Geometry check sheet. Reference: the model listing, model coordinates, mm. Face numbers are marked on the shaded views. A direction names the side the tool comes from. Round coordinates to 2 decimals unless told otherwise and drop trailing zeros. Write each loop counter-clockwise with the first axis right and the second up, starting at its lowest first coordinate (ties: lowest second). Pieces come first, ordered by that corner, then holes. Notation, with made-up numbers: M -10.5,56.25 L 5.5,56.25 A20 ccw 5.5,94.25 Z; hole C 63,-34.75 d6. An arc over 180 degrees is marked long. Answer as CSV lines item,"result". Start each with the question number.
```python
from build123d import *

# Parameters (mm, degrees)
SKETCH1_R               = 3.175
SKETCH1_R_2             = 2.38125
BOSS_EXTRUDE1_DEPTH     = 2.794
SKETCH2_R               = 4.7625
SKETCH2_R_2             = 2.38125
BOSS_EXTRUDE2_DEPTH     = 1.6256
SKETCH3_R               = 22.361166229
SKETCH3_R_2             = 11.176
CUT_EXTRUDE1_DEPTH      = 5.7625
CUT_EXTRUDE1_DEPTH_BACK = 5.7625
SKETCH4_W               = 0.762
SKETCH4_H               = 2.54
CUT_EXTRUDE2_DEPTH      = 5.7625001
CUT_EXTRUDE2_DEPTH_BACK = 5.7625001


with BuildPart() as part:
    # Sketch1 → Boss-Extrude1 (new body)
    with BuildSketch(Plane.XY):
        Circle(SKETCH1_R)
        Circle(SKETCH1_R_2, mode=Mode.SUBTRACT)
    extrude(amount=BOSS_EXTRUDE1_DEPTH)

    # Sketch2 → Boss-Extrude2 (add)
    with BuildSketch(Plane.XY.offset(2.794)):
        Circle(SKETCH2_R)
        Circle(SKETCH2_R_2, mode=Mode.SUBTRACT)
    extrude(amount=BOSS_EXTRUDE2_DEPTH)

    # Sketch3 → Cut-Extrude1 (cut, two sides)
    with BuildSketch(Plane(origin=(0, 0, 0), x_dir=(0, 0, -1), z_dir=(1, 0, 0))) as cut_extrude1_sk:
        with Locations((6.7564, 0)):
            Circle(SKETCH3_R)
        with Locations((6.7564, 0)):
            Circle(SKETCH3_R_2, mode=Mode.SUBTRACT)
    extrude(amount=CUT_EXTRUDE1_DEPTH, mode=Mode.SUBTRACT)
    extrude(cut_extrude1_sk.sketch, amount=-CUT_EXTRUDE1_DEPTH_BACK, mode=Mode.SUBTRACT)

    # Sketch4 → Cut-Extrude2 (cut, two sides)
    with BuildSketch(Plane(origin=(0, 0, 0), x_dir=(0, 0, -1), z_dir=(1, 0, 0))) as cut_extrude2_sk:
        with Locations((-4.0386, 0)):
            Rectangle(SKETCH4_W, SKETCH4_H)
    extrude(amount=CUT_EXTRUDE2_DEPTH, mode=Mode.SUBTRACT)
    extrude(cut_extrude2_sk.sketch, amount=-CUT_EXTRUDE2_DEPTH_BACK, mode=Mode.SUBTRACT)


solid = part.part
```
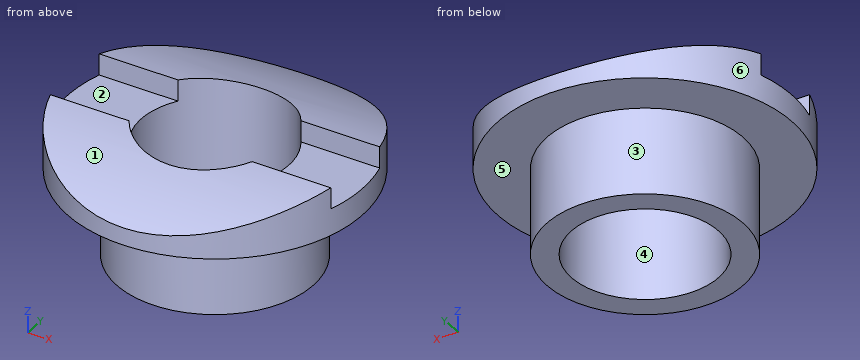
1) Section check D-D, the plane x = 3.75. Record the cut outline in (y, z).
2) Scan lines: line 1 (Y direction, x = 0, z = 2.05) (3 decimals); line 2 (X direction, y = -0.5, z = 3); line 3 (X direction, y = -0.75, z = 0.8). Record each from-to range of solid material in increasing order. Write a range as from..to.
3) Section check B-B, the plane x = 0. Record the cut outline in (y, z) (1 decimal).
4) Access from +Z, -Z, +X, -X, +Y, -Y to the whole of each face (thin tool, end or side, straight path). Record for the marked faces 1, 2 and 3.
5) Mould release check, pull along X, two halves, no side actions. Record for the marked faces 4, 5 and 6: released by +X, released by -X, zero draft, split by the parting line, or undercut.
6) Go/stop test with flat-tipped pins: pin 1 (1 mm diameter, centred on y = 2.5, z = 1.5, fed in from +X); pin 2 (2 mm diameter, centred on x = 3.5, y = 0, fed in from +Z); pin 3 (1 mm diameter, centred on x = 0.5, z = 2, fed in from +Y) (3 decimals). Record where each tip stops, or that it passes through.
7) Section check A-A, the plane y = 0. Record the cut outline in (x, z) (1 decimal), plus the area to 3 significant figures.
Results:
1,outline,"M -2.94,2.79 L 2.94,2.79 L 2.94,4.03 A11.18 ccw 1.27,4.35 L 1.27,3.66 L -1.27,3.66 L -1.27,4.35 A11.18 ccw -2.94,4.03 Z"
2,line 1,"y = -3.175..-2.381, 2.381..3.175"
2,line 2,"x = -4.74..-2.33, 2.33..4.74"
2,line 3,"x = -3.09..-2.26, 2.26..3.09"
3,outline,"M -4.8,2.8 L -3.2,2.8 L -3.2,0 L -2.4,0 L -2.4,4.2 A11.2 ccw -4.8,3.4 Z; M 2.4,0 L 3.2,0 L 3.2,2.8 L 4.8,2.8 L 4.8,3.4 A11.2 ccw 2.4,4.2 Z"
4,face 1,"+Z, +X, -X, -Y"
4,face 2,"+Z, +X, -X"
4,face 3,"-Z"
5,face 4,"undercut"
5,face 5,"zero draft"
5,face 6,"split by the parting line"
6,pin 1,"stops at x = 2.47"
6,pin 2,"stops at z = 3.66"
6,pin 3,"stops at y = 3.175"
7,outline,"M -4.8,2.8 L -3.2,2.8 L -3.2,0 L -2.4,0 L -2.4,3.7 L -4.8,3.7 Z; M 2.4,0 L 3.2,0 L 3.2,2.8 L 4.8,2.8 L 4.8,3.7 L 2.4,3.7 Z"
7,area,"8.55 mm^2"
